Part print with two shaded views. Sizes in mm from the minimum x, y, z corner. A direction names the side the tool comes from. Round coordinates to 2 decimals unless told otherwise and drop trailing zeros. Loops run counter-clockwise (first coordinate to the right, second up) from the corner with the lowest first, then second, coordinate; pieces in that order, holes last.
(1) Mould opens along Y. For the marked faces 1, 2 and 3 say: +Y half, -Y half, draft (parallel to the pull), parting line (faces both ways), or undercut.
(2) Cut at A-A on x = 12.5. List the corners of the cut face in (y, z).
(3) Cut at C-C on z = 3.15. List the corners of the cut face in (x, y).
(4) Probe probe 1 along Y at (x, z) = (1.75, 1.9); probe 2 along Y at (x, z) = (9.5, 0.3); probe 3 along Y at (x, z) = (7.75, 0.7). List the from-to ranges inside material, lowest first.
(5) Cut at D-D on x = 10.25. List the corners of the cut face in (y, z).
(6) Flat gauge pins, fed straight in: pin 1 (1.6 mm diameter, centred on y = 12, z = 0.5, fed in from -X); pin 2 (1 mm diameter, centred on y = 19, z = 1.5, fed in from -X); pin 3 (1 mm diameter, centred on y = 12.5, z = 0.5, fed in from +X). Where does each tip first touch, or does it go through?
(7) Cut at B-B on y = 5.75. List the corners of the cut face in (x, z), then the cut area to 3 significant figures.
(8) Tool access for the marked faces 4, 5 and 6: list every direction of +Z, -Z, +X, -X, +Y, -Y with a clear straight run to the whole face (end or side of a thin tool).
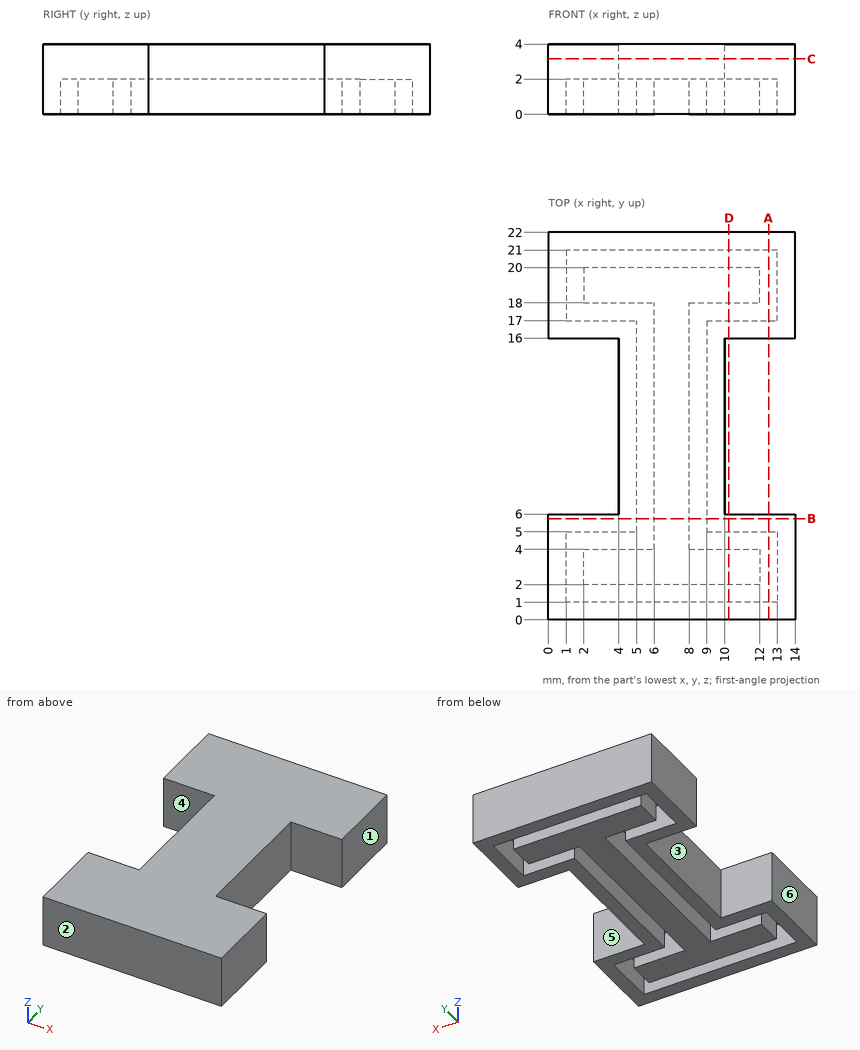
Final values:
1. face 1: draft
1. face 2: -Y half
1. face 3: undercut
2. outline: (0, 0) - (1, 0) - (1, 2) - (5, 2) - (5, 0) - (6, 0) - (6, 4) - (0, 4) - close; (16, 0) - (17, 0) - (17, 2) - (21, 2) - (21, 0) - (22, 0) - (22, 4) - (16, 4) - close
3. outline: (0, 0) - (14, 0) - (14, 6) - (10, 6) - (10, 16) - (14, 16) - (14, 22) - (0, 22) - (0, 16) - (4, 16) - (4, 6) - (0, 6) - close
4. probe 1: y = 0 to 1, 5 to 6, 16 to 17, 21 to 22
4. probe 2: y = 0 to 1, 2 to 4, 5 to 17, 18 to 20, 21 to 22
4. probe 3: y = 0 to 1, 2 to 20, 21 to 22
5. outline: (0, 0) - (1, 0) - (1, 2) - (2, 2) - (2, 0) - (4, 0) - (4, 2) - (5, 2) - (5, 0) - (6, 0) - (6, 4) - (0, 4) - close; (16, 0) - (17, 0) - (17, 2) - (18, 2) - (18, 0) - (20, 0) - (20, 2) - (21, 2) - (21, 0) - (22, 0) - (22, 4) - (16, 4) - close
6. pin 1: stops at x = 4
6. pin 2: stops at x = 0
6. pin 3: stops at x = 10
7. outline: (0, 0) - (5, 0) - (5, 2) - (6, 2) - (6, 0) - (8, 0) - (8, 2) - (9, 2) - (9, 0) - (14, 0) - (14, 4) - (0, 4) - close
7. area: 52.0 mm2
8. face 4: +Z, -Z, -X
8. face 5: +Z, -Z, +X
8. face 6: +Z, -Z, -X, +Y, -Y
